Can you work these out from the model? Positions are in its coordinate system, mm. A direction names the side the tool comes from. Round coordinates to 2 decimals unless told otherwise and drop trailing zeros. Write each loop counter-clockwise with the first axis right and the second up, starting at its lowest first coordinate (ties: lowest second). Pieces come first, ordered by that corner, then holes.
Q1. Please list where these lines run through material, in increasing order: line 1 along Z through (x, y) = (43, 0.5); line 2 along X through (y, z) = (4.5, 11); line 3 along Z through (x, y) = (-1, 1.75).
Q2. I'm going to push flat-ended pins straight in: pin 1 Ø3 at (x, z) = (30, 81.5) entering from +Y; pin 2 Ø1.5 at (x, y) = (13, 4) entering from +Z; pin 3 Ø12 at (x, z) = (-11.5, -5.5) entering from +Y. Where does each tip first touch, or does it pass through?
Q3. If we section it at B-B (y = 4.75): Please give me the cut outline in (x, z), plus the area to 3 significant figures.
Q4. We'd pull the mould along X, two halves only. Please class faces 3 (the flat face through (-90, 5, 1)), 4 (the flat face through (90, 5, 1)), 5 (the flat face through (-1, 1, 70)), 6 (the flat face through (-7, 1, -82.5)): +X half, -X half, draft (parallel to the pull), parting line (faces both ways), or undercut.
Q5. If we section it at A-A (x = -23): Please give me the cut outline in (y, z), plus the area to 3 significant figures.
Q6. If we section it at C-C (z = 4.5): Please give me the cut outline in (x, y).
Q7. If we section it at D-D (z = 43.5): Please give me the cut outline in (x, y), plus the area to 3 significant figures.
Q8. For faces 1 (the flat face through (-1, 1, -70)), 2 (the flat face through (85, 10, -1)), which set-ups out of +Z, -Z, +X, -X, +Y, -Y let a thin tool reach every point of the face, with its end or its side?
from build123d import *

# Parameters (mm, degrees)
SKETCH5_W           = 180
SKETCH5_H           = 165
SKETCH5_W_2         = 160
SKETCH5_H_2         = 40
BOSS_EXTRUDE3_DEPTH = 1
SKETCH6_W           = 10
SKETCH6_H           = 165
BOSS_EXTRUDE4_DEPTH = 9
SKETCH7_W           = 160
SKETCH7_H           = 2.5
BOSS_EXTRUDE5_DEPTH = 1
SKETCH10_W          = 160
SKETCH10_H          = 2.5
BOSS_EXTRUDE6_DEPTH = 1


with BuildPart() as part:
    # Sketch5 → Boss-Extrude3 (new body)
    with BuildSketch(Plane(origin=(0, 0, 0), x_dir=(1, 0, 0), z_dir=(0, 1, 0))):
        Rectangle(SKETCH5_W, SKETCH5_H)
        with Locations((0, -40)):
            Rectangle(SKETCH5_W_2, SKETCH5_H_2, mode=Mode.SUBTRACT)
        with Locations((0, 40)):
            Rectangle(SKETCH5_W_2, SKETCH5_H_2, mode=Mode.SUBTRACT)
    extrude(amount=BOSS_EXTRUDE3_DEPTH)

    # Sketch6 → Boss-Extrude4 (add)
    with BuildSketch(Plane(origin=(0, 1, 0), x_dir=(1, 0, 0), z_dir=(0, 1, 0))):
        with Locations((-85, 0)):
            Rectangle(SKETCH6_W, SKETCH6_H)
        with Locations((85, 0)):
            Rectangle(SKETCH6_W, SKETCH6_H)
    extrude(amount=BOSS_EXTRUDE4_DEPTH)

    # Sketch7 → Boss-Extrude5 (add)
    with BuildSketch(Plane(origin=(0, 1, 0), x_dir=(1, 0, 0), z_dir=(0, 1, 0))):
        with Locations((0, -81.25)):
            Rectangle(SKETCH7_W, SKETCH7_H)
    extrude(amount=BOSS_EXTRUDE5_DEPTH)

    # Sketch10 → Boss-Extrude6 (add)
    with BuildSketch(Plane(origin=(0, 1, 0), x_dir=(1, 0, 0), z_dir=(0, 1, 0))):
        with Locations((0, 81.25)):
            Rectangle(SKETCH10_W, SKETCH10_H)
    extrude(amount=BOSS_EXTRUDE6_DEPTH)


solid = part.part
A:
1. line 1: z = -82.5 to -60, -20 to 20, 60 to 82.5
1. line 2: x = -90 to -80, 80 to 90
1. line 3: z = -82.5 to -80, 80 to 82.5
2. pin 1: stops at y = 2
2. pin 2: passes through
2. pin 3: stops at y = 1
3. outline: (-90, -82.5) - (-80, -82.5) - (-80, 82.5) - (-90, 82.5) - close; (80, -82.5) - (90, -82.5) - (90, 82.5) - (80, 82.5) - close
3. area: 3,300 mm2
4. face 3: -X half
4. face 4: +X half
4. face 5: undercut
4. face 6: draft
5. outline: (0, -82.5) - (2, -82.5) - (2, -80) - (1, -80) - (1, -60) - (0, -60) - close; (0, -20) - (1, -20) - (1, 20) - (0, 20) - close; (0, 60) - (1, 60) - (1, 80) - (2, 80) - (2, 82.5) - (0, 82.5) - close
5. area: 90.0 mm2
6. outline: (-90, 0) - (90, 0) - (90, 10) - (80, 10) - (80, 1) - (-80, 1) - (-80, 10) - (-90, 10) - close
7. outline: (-90, 0) - (-80, 0) - (-80, 10) - (-90, 10) - close; (80, 0) - (90, 0) - (90, 10) - (80, 10) - close
7. area: 200 mm2
8. face 1: +Y
8. face 2: +Z, -Z, +X, -X, +Y
